from build123d import *

# Parameters (mm, degrees)
F0_W     = 900
F0_H     = 650
F1_DEPTH = 300
F3_DEPTH = 300
F4_W     = 300
F4_H     = 250
F5_DEPTH = 300.001


with BuildPart() as f1:
    # F0 (on Front) → F1 (new body)
    with BuildSketch(Plane.XZ):
        Rectangle(F0_W, F0_H)
    extrude(amount=F1_DEPTH)

    # F2 (on face) → F3 (join)
    with BuildSketch(Plane.XZ.offset(300)):
        Polygon((450, -325), (450, 325), (227.090806, -325), align=None)
        Polygon((-214.815646, -325), (-450, 325), (-450, -325), align=None)
    extrude(amount=F3_DEPTH)

    # F4 (on face) → F5 (cut, through all)
    with BuildSketch(Plane.XZ.offset(300)):
        with Locations((5.15289, 200)):
            Rectangle(F4_W, F4_H)
    extrude(amount=-F5_DEPTH, mode=Mode.SUBTRACT)


solid = f1.part
The listing builds one solid part. Answer for the finished solid, in the listing's coordinates (mm). A direction names the side the tool comes from. Give positions to 0.01 mm unless a question says otherwise; leave off trailing zeros. Loops run counter-clockwise (first coordinate to the right, second up) from the corner with the lowest first, then second, coordinate; pieces in that order, holes last. Notation, with made-up numbers: (24, 26) - (40, 26) arc R16 ccw to (40, 49) - close; hole circle Ø7 at (-8.75, 41.25). An arc over 180 degrees is marked (long way). Write each question's results on one line, items separated by ' | '.
1. Which of the six approach directions +Z, -Z, +X, -X, +Y, -Y give full straight-line access (tool end or side, diameter ignored) to faces 4 (the face through (-144.847, -152, 198)), 5 (the face through (340.106, -447.9, 4.55)), 6 (the face through (387, -600, -140))?
Resolved:
face 4: +Z, +Y, -Y | face 5: +Z, -Y | face 6: +Z, -Z, +X, -X, -Y
2. Flat-ended cylindrical pins translate along their axes: P1, Ø1.5, axis at x = 348.5, z = 111.5, coming from the -Y side; P2, Ø5, axis at x = -340.5, z = -236, coming from the +Y side. Find the tip coordinate at first contact, or state that the pin passes through.
Resolved:
P1: stops at y = -300 | P2: stops at y = 0
3. Find section A-A, the plane z = 136. Write down the section's boundary in (x, y).
Resolved:
outline: (-450, -600) - (-381.62, -600) - (-381.62, -300) - (-144.85, -300) - (-144.85, 0) - (-450, 0) - close; (155.15, -300) - (385.18, -300) - (385.18, -600) - (450, -600) - (450, 0) - (155.15, 0) - close
4. Consider probe 1 along Z at (x, y) = (18, -252.5); probe 2 along X at (y, z) = (-159, 161.5); probe 3 along X at (y, z) = (-314, 271.5). Determine where each line is inside the solid, lowest interval first. Write a range as from..to.
Resolved:
probe 1: z = -325..75 | probe 2: x = -450..-144.85, 155.15..450 | probe 3: x = -450..-430.64, 431.65..450
5. For a pull along X with two mould halves and no side action, classify faces 1 (the face through (-386, -600, -140)), 2 (the face through (-6, -300, 5)), 3 (the face through (-450, -296, -5)) as +X half, -X half, draft (parallel to the pull), parting line (faces both ways), or undercut.
Resolved:
face 1: draft | face 2: undercut | face 3: -X half
6. Find section C-C, the plane y = -206. Write down the section's boundary in (x, z), then the cut area to 3 significant figures.
Resolved:
outline: (-450, -325) - (450, -325) - (450, 325) - (155.15, 325) - (155.15, 75) - (-144.85, 75) - (-144.85, 325) - (-450, 325) - close | area: 510,000 mm^2
7. Find section D-D, the plane x = -45. Write down the section's boundary in (y, z), then the cut area to 3 significant figures.
Resolved:
outline: (-300, -325) - (0, -325) - (0, 75) - (-300, 75) - close | area: 120,000 mm^2
8. Find section B-B, the plane y = -484.5. Write down the section's boundary in (x, z).
Resolved:
outline: (-450, -325) - (-214.82, -325) - (-450, 325) - close; (227.09, -325) - (450, -325) - (450, 325) - close
